Geometry: final body of the model. Coordinates: model frame, mm. A direction names the side the tool comes from. Coordinates: 2 decimals unless noted, no trailing zeros. Write each loop counter-clockwise with the first axis right and the second up, starting at its lowest first coordinate (ties: lowest second). Pieces come first, ordered by that corner, then holes. Notation, with made-up numbers: M 77.5,66 L 117.5,66 A8 ccw 117.5,81 Z; hole C 41.5,-13.75 d2. An arc over 180 degrees is marked long. Write item = value, one per line. Start each with the question number.
Item 1: First-contact query: pin 1 Ø1 at (x, z) = (-7.46, -14.6) entering from -Y; pin 2 Ø3 at (x, y) = (2.5, 4) entering from +Z; pin 3 Ø2 at (x, z) = (-1.5, -7) entering from +Y; pin 4 Ø3 at (x, y) = (1.5, 10) entering from -Z. Flat tips, straight axial feed; report the tip coordinate or a pass-through.
Item 2: Section B-B on y = 4.5. Output: boundary loops of the cut face in (x, z).
Item 3: Section D-D on z = -4.5. Output: boundary loops of the cut face in (x, y), plus the area to 3 significant figures.
Item 4: Section A-A on y = 22.5. Output: boundary loops of the cut face in (x, z).
Item 5: Section C-C on x = -4. Output: boundary loops of the cut face in (y, z).
Item 6: Ray query, L1, parallel to Y at x = -4.5, z = 15.5; L2, parallel to X at y = 10, z = -7.5; L3, parallel to Y at x = 7.5, z = 7. Return the intervals inside material, ascending. Write a range as [from, to].
Item 7: Reachability of faces 5 (the flat face through (-6, 8, 0)), 6 (the flat face through (0, 18, 14)), 7 (the cylindrical face through (-5.715, 7.888, -12.199)), 8 (the cylindrical face through (-5.699, 7.888, 12.215)) from +Z, -Z, +X, -X, +Y, -Y: full face, straight path, thin tool, end or side. Return the list, or none.
Item 8: Pull-direction query (Z, two-part tool) for faces 1 (the flat face through (0, 25, 8)), 2 (the flat face through (0, 8, -12.5)), 3 (the flat face through (0, 20, 12.5)), 4 (the cylindrical face through (-8.013, 17.014, -14.31)); classes: +Z half, -Z half, draft (parallel to the pull), parting line (faces both ways), or undercut.
from build123d import *

# Parameters (mm, degrees)
BOSS_EXTRUDE1_DEPTH = 16
BOSS_EXTRUDE2_DEPTH = 2
BOSS_EXTRUDE3_DEPTH = 9
SKETCH5_R           = 0.622765991
CUT_EXTRUDE1_DEPTH  = 18
FILLET1_R           = 0.1
SKETCH6_R           = 3
SKETCH6_R_2         = 2
BOSS_EXTRUDE4_DEPTH = 1
BOSS_EXTRUDE5_DEPTH = 3


with BuildPart() as part:
    # Sketch1 → Boss-Extrude1 (new body)
    with BuildSketch(Plane(origin=(0, 0, 0), x_dir=(1, 0, 0), z_dir=(0, 1, 0))):
        with BuildLine():
            Line((-5, 12.5), (5, 12.5))
            ThreePointArc((5, 12.5), (5.707106781, 12.207106781), (6, 11.5))
            Line((6, 11.5), (6, -11.5))
            ThreePointArc((6, -11.5), (5.707106781, -12.207106781), (5, -12.5))
            Line((5, -12.5), (-5, -12.5))
            ThreePointArc((-5, -12.5), (-5.707106781, -12.207106781), (-6, -11.5))
            Line((-6, -11.5), (-6, 11.5))
            ThreePointArc((-6, 11.5), (-5.707106781, 12.207106781), (-5, 12.5))
        make_face()
    extrude(amount=BOSS_EXTRUDE1_DEPTH)

    # Sketch2 → Boss-Extrude2 (add)
    with BuildSketch(Plane(origin=(0, 16, 0), x_dir=(1, 0, 0), z_dir=(0, 1, 0))):
        with BuildLine():
            Line((-8, 16), (8, 16))
            ThreePointArc((8, 16), (8.707106781, 15.707106781), (9, 15))
            Line((9, 15), (9, -15))
            ThreePointArc((9, -15), (8.707106781, -15.707106781), (8, -16))
            Line((8, -16), (-8, -16))
            ThreePointArc((-8, -16), (-8.707106781, -15.707106781), (-9, -15))
            Line((-9, -15), (-9, 15))
            ThreePointArc((-9, 15), (-8.707106781, 15.707106781), (-8, 16))
        make_face()
    extrude(amount=BOSS_EXTRUDE2_DEPTH)

    # Sketch4 → Boss-Extrude3 (add, symmetric)
    with BuildSketch(Plane(origin=(0, 0, 0), x_dir=(0, 0, -1), z_dir=(1, 0, 0))):
        with BuildLine():
            Line((-12.5, 18), (13.5, 18))
            ThreePointArc((13.5, 18), (10.126897029, 19.440345543), (7.5, 22))
            Line((7.5, 22), (-12.5, 22))
            Line((-12.5, 22), (-12.5, 18))
        make_face()
    extrude(amount=BOSS_EXTRUDE3_DEPTH, both=True)

    # Sketch5 → Cut-Extrude1 (cut)
    with BuildSketch(Plane(origin=(0, 18, 0), x_dir=(1, 0, 0), z_dir=(0, 1, 0))):
        with Locations(Location((-7.460775455, -14.595038574, 0), (0, 0, 270))):
            Circle(SKETCH5_R)
        with Locations(Location((7.561200473, -14.595038574, 0), (0, 0, 270))):
            Circle(SKETCH5_R)
        with Locations(Location((-7.460775455, 14.59721935, 0), (0, 0, 270))):
            Circle(SKETCH5_R)
        with Locations(Location((7.561200473, 14.59721935, 0), (0, 0, 270))):
            Circle(SKETCH5_R)
    extrude(amount=-CUT_EXTRUDE1_DEPTH, mode=Mode.SUBTRACT)

    # Fillet1
    fillet1_edges = [part.edges().sort_by_distance(p)[0] for p in [
        (-9, 20, 12.5),
        (0, 22, 12.5),
        (-9, 19.440345543, -10.126897029),
        (-9, 22, 2.5),
        (0, 22, -7.5),
        (9, 20, 12.5),
        (9, 19.440345543, -10.126897029),
        (9, 22, 2.5),
    ]]
    fillet(fillet1_edges, radius=FILLET1_R)

    # Sketch6 → Boss-Extrude4 (add)
    with BuildSketch(Plane(origin=(0, 22, 0), x_dir=(1, 0, 0), z_dir=(0, 1, 0))):
        with Locations(Location((0, -8, 0), (0, 0, 90))):
            Circle(SKETCH6_R)
        with Locations(Location((0, -8, 0), (0, 0, 270))):
            Circle(SKETCH6_R_2, mode=Mode.SUBTRACT)
    extrude(amount=BOSS_EXTRUDE4_DEPTH)

    # Sketch7 → Boss-Extrude5 (add)
    with BuildSketch(Plane(origin=(0, 22, 0), x_dir=(1, 0, 0), z_dir=(0, 1, 0))):
        Polygon((-1.117847018, -6.882152982), (-1.460537515, -7.395025553), (-1.580874414, -8), (-1.460537515, -8.604974447), (-1.117847018, -9.117847018), (-0.604974447, -9.460537515), (0, -9.580874414), (0.604974447, -9.460537515), (1.117847018, -9.117847018), (1.460537515, -8.604974447), (1.580874414, -8), (1.460537515, -7.395025553), (1.117847018, -6.882152982), (0.604974447, -6.539462485), (0, -6.419125586), (-0.604974447, -6.539462485), align=None)
    extrude(amount=BOSS_EXTRUDE5_DEPTH)


solid = part.part
Responses:
q1.pin_1 = through
q1.pin_2 = 12.5
q1.pin_3 = 22
q1.pin_4 = -12.5
q2.outline = M -6,-11.5 A1 ccw -5,-12.5 L 5,-12.5 A1 ccw 6,-11.5 L 6,11.5 A1 ccw 5,12.5 L -5,12.5 A1 ccw -6,11.5 Z
q3.outline = M -9,16 L -6,16 L -6,0 L 6,0 L 6,16 L 9,16 L 9,21.9 A0.1 ccw 8.9,22 L -8.9,22 A0.1 ccw -9,21.9 Z
q3.area = 300 mm²
q4.outline = C 0,8 d6; M -1.58,8 L -1.46,7.4 L -1.12,6.88 L -0.6,6.54 L 0,6.42 L 0.6,6.54 L 1.12,6.88 L 1.46,7.4 L 1.58,8 L 1.46,8.6 L 1.12,9.12 L 0.6,9.46 L 0,9.58 L -0.6,9.46 L -1.12,9.12 L -1.46,8.6 Z; hole C 0,8 d4
q5.outline = M 0,-12.5 L 16,-12.5 L 16,-16 L 18,-16 L 18,-13.5 A10 cw 21.96,-7.53 A0.1 ccw 22,-7.45 L 22,12.4 A0.1 ccw 21.9,12.5 L 18,12.5 L 18,16 L 16,16 L 16,12.5 L 0,12.5 Z
q6.L1 = [16, 18]
q6.L2 = [-6, 6]
q6.L3 = [16, 22]
q7.face_5 = +Z, -Z, -X, -Y
q7.face_6 = +Z, +X, -X, +Y
q7.face_7 = -Z, -X, -Y
q7.face_8 = +Z, -X, -Y
q8.face_1 = draft
q8.face_2 = -Z half
q8.face_3 = +Z half
q8.face_4 = undercut
